Build history of the part. All positions in model axes, mm. Round coordinates to 2 decimals unless told otherwise and drop trailing zeros. Loops run counter-clockwise (first coordinate to the right, second up) from the corner with the lowest first, then second, coordinate; pieces in that order, holes last. Notation, with made-up numbers: (71, 78) - (96, 78) arc R36 cw to (96, 116) - close; hole circle Ø10 at (26, -25). An arc over 180 degrees is marked (long way). Use a Markdown table: item, result.
from build123d import *

# Parameters (mm, degrees)
DODANIE_WYCI_GNI_CIE1_DEPTH   = 110
DODANIE_WYCI_GNI_CIE1_2_DEPTH = 110
SZKIC2_W                      = 45
SZKIC2_H                      = 5
DODANIE_WYCI_GNI_CIE2_DEPTH   = 4
SZKIC4_W                      = 35
SZKIC4_H                      = 30
WYTNIJ_WYCI_GNI_CIE1_DEPTH    = 10
SZKIC5_W                      = 45
SZKIC5_H                      = 50
DODANIE_WYCI_GNI_CIE3_DEPTH   = 4
SZKIC6_W                      = 4
SZKIC6_H                      = 148
WYTNIJ_WYCI_GNI_CIE2_DEPTH    = 10
SFAZOWANIE1_SIZE              = 4
DODANIE_WYCI_GNI_CIE4_DEPTH   = 2
SZKIC9_W                      = 15
SZKIC9_H                      = 45
WYTNIJ_WYCI_GNI_CIE3_DEPTH    = 80


with BuildPart() as part:
    # Szkic1 → Dodanie-wyci_gni_cie1 (new body)
    with BuildSketch(Plane.XY):
        Polygon((-7.5, -2), (-11.5, 2), (-22.5, 2), (-22.5, -2), align=None)
    extrude(amount=-DODANIE_WYCI_GNI_CIE1_DEPTH)



with BuildPart() as body_2:
    # Szkic1 → Dodanie-wyci_gni_cie1 2 (new body)
    with BuildSketch(Plane.XY):
        Polygon((22.5, 2), (11.5, 2), (7.5, -2), (22.5, -2), align=None)
    extrude(amount=-DODANIE_WYCI_GNI_CIE1_2_DEPTH)


with BuildPart() as part_1:
    add(part.part)

    add(body_2.part)  # Dodanie-wyci_gni_cie2 merges body 2
    # Szkic2 → Dodanie-wyci_gni_cie2 (add)
    with BuildSketch(Plane.XZ.offset(2)):
        with Locations((0, 2.5)):
            Rectangle(SZKIC2_W, SZKIC2_H)
        with Locations((0, -112.5)):
            Rectangle(SZKIC2_W, SZKIC2_H)
    extrude(amount=-DODANIE_WYCI_GNI_CIE2_DEPTH)

    # Szkic4 → Wytnij-wyci_gni_cie1 (cut)
    with BuildSketch(Plane(origin=(0, 2, 0), x_dir=(1, 0, 0), z_dir=(0, 1, 0))):
        with Locations((22.5, 55)):
            Rectangle(SZKIC4_W, SZKIC4_H)
    extrude(amount=-WYTNIJ_WYCI_GNI_CIE1_DEPTH, mode=Mode.SUBTRACT)

    # Szkic5 → Dodanie-wyci_gni_cie3 (add)
    with BuildSketch(Plane.XZ.offset(2)):
        with Locations((0, -140)):
            Rectangle(SZKIC5_W, SZKIC5_H)
        Polygon((37.5, 5), (22.5, 5), (22.5, -40), (22.5, -70), (22.5, -115), (22.5, -165), (37.5, -165), align=None)
    extrude(amount=-DODANIE_WYCI_GNI_CIE3_DEPTH)

    # Szkic6 → Wytnij-wyci_gni_cie2 (cut)
    with BuildSketch(Plane(origin=(0, 2, 0), x_dir=(1, 0, 0), z_dir=(0, 1, 0))):
        with Locations((24.5, 81)):
            Rectangle(SZKIC6_W, SZKIC6_H)
    extrude(amount=-WYTNIJ_WYCI_GNI_CIE2_DEPTH, mode=Mode.SUBTRACT)

    # Sfazowanie1
    sfazowanie1_edges = [part_1.edges().sort_by_distance(p)[0] for p in [
        (22.5, 2, -23.5),
        (22.5, 2, -112.5),
        (26.5, 2, -81),
    ]]
    chamfer(sfazowanie1_edges, length=SFAZOWANIE1_SIZE - 0.0001)  # a hair under: the kernel refuses the full size

    # Szkic7 → Dodanie-wyci_gni_cie4 (add)
    with BuildSketch(Plane(origin=(0, 0, 0), x_dir=(-1, 0, 0), z_dir=(0, 0, -1))):
        Polygon((-11.5, 2), (-7.5, -2), (7.5, -2), (11.5, 2), align=None)
    extrude(amount=DODANIE_WYCI_GNI_CIE4_DEPTH)

    # Szkic9 → Wytnij-wyci_gni_cie3 (cut)
    with BuildSketch(Plane.XZ.offset(2)):
        with Locations((15, -54.5)):
            Rectangle(SZKIC9_W, SZKIC9_H)
    extrude(amount=-WYTNIJ_WYCI_GNI_CIE3_DEPTH, mode=Mode.SUBTRACT)


solid = part_1.part
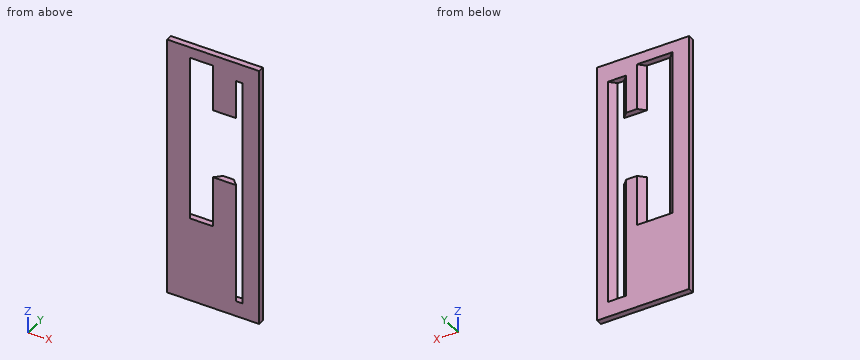
Q1. Cut at D-D, the plane y = 0.45. List the corners of the cut face in (x, z), plus the area to 3 significant figures.
Results found:
| item | result |
|---|---|
| outline | (-22.5, -165) - (37.5, -165) - (37.5, 5) - (-22.5, 5) - close; hole (-9.95, -110) - (9.95, -110) - (9.95, -77) - (20.05, -77) - (20.05, -155) - (28.95, -155) - (28.95, -7) - (20.05, -7) - (20.05, -32) - (9.95, -32) - (9.95, -2) - (-9.95, -2) - close |
| area | 6,280 mm2 |
Q2. Probe line 1 (X direction, y = 1.35, z = -100); line 2 (Z direction, x = 20.5, y = -0.75); line 3 (X direction, y = 1.65, z = -12). List the from-to ranges inside material, lowest first.
Results found:
| item | result |
|---|---|
| line 1 | x = -22.5 to -10.85, 10.85 to 19.15, 29.85 to 37.5 |
| line 2 | z = -165 to -77, -32 to 5 |
| line 3 | x = -22.5 to -11.15, 11.15 to 18.85, 30.15 to 37.5 |
Q3. Cut at A-A, the plane x = 15. List the corners of the cut face in (y, z).
Results found:
| item | result |
|---|---|
| outline | (-2, -165) - (2, -165) - (2, -77) - (-2, -77) - close; (-2, -32) - (2, -32) - (2, 5) - (-2, 5) - close |
Q4. Cut at B-B, the plane z = -12. Count the separate pieces of the cut face and the enclosed holes in it, plus the area to 3 significant figures.
Results found:
| item | result |
|---|---|
| separate pieces | 3 |
| enclosed holes | 0 |
| area | 132 mm2 |
